Source: CAD feature listing. Evaluate the final solid. Frame: model axes, mm. Give positions to 0.01 mm unless a question says otherwise; leave off trailing zeros. Order: outer loops, then holes, each group sorted by start corner. A loop starts at its lowest first (then second) coordinate and runs counter-clockwise, first axis right, second up. Notation, with made-up numbers: (-5.75, -7.5) - (9.25, -7.5) arc R18 ccw to (9.25, 1.5) - close; hole circle Ø1 at (46, 44). An arc over 180 degrees is marked (long way). Use CSV: the item, a comma, the result in double quotes.
```python
from build123d import *

# Parameters (mm, degrees)
SKETCH_1_W          = 70
SKETCH_1_H          = 133.34
EXTRUDE_1_DEPTH     = 1.6
SKETCH_2_R          = 1.5
SKETCH_2_W          = 18
SKETCH_2_H          = 1
SKETCH_2_W_2        = 17.5
SKETCH_2_W_3        = 7.5
CUT_EXTRUDE_1_DEPTH = 76.315661718
FILLET_1_R          = 3
FILLET_2_R          = 0.5


with BuildPart() as part:
    # ｽｹｯﾁ1 → ﾎﾞｽ - 押し出し1 (new body)
    with BuildSketch(Plane(origin=(0, 0, 0), x_dir=(1, 0, 0), z_dir=(0, 1, 0))):
        Rectangle(SKETCH_1_W, SKETCH_1_H)
    extrude(amount=EXTRUDE_1_DEPTH)

    # ｽｹｯﾁ2 → ｶｯﾄ - 押し出し1 (cut, through all)
    with BuildSketch(Plane(origin=(0, 1.6, 0), x_dir=(1, 0, 0), z_dir=(0, 1, 0))):
        with Locations(Location((-22.86, -37.46, 0), (0, 0, 270))):
            Circle(SKETCH_2_R)
        with Locations(Location((22.86, -37.46, 0), (0, 0, 90))):
            Circle(SKETCH_2_R)
        with Locations(Location((-24.13, 41.65, 0), (0, 0, 270))):
            Circle(SKETCH_2_R)
        with Locations(Location((24.13, 39.95, 0), (0, 0, 270))):
            Circle(SKETCH_2_R)
        with Locations(Location((8.89, -10.85, 0), (0, 0, 270))):
            Circle(SKETCH_2_R)
        with Locations((-26, 44.15)):
            Rectangle(SKETCH_2_W, SKETCH_2_H)
        with Locations((26, 44.15)):
            Rectangle(SKETCH_2_W, SKETCH_2_H)
        with Locations((-5.25, 44.15)):
            Rectangle(SKETCH_2_W_2, SKETCH_2_H)
        with Locations((10.25, 44.15)):
            Rectangle(SKETCH_2_W_3, SKETCH_2_H)
    extrude(amount=-CUT_EXTRUDE_1_DEPTH, mode=Mode.SUBTRACT)

    # ﾌｨﾚｯﾄ1
    fillet_1_edges = [part.edges().sort_by_distance(p)[0] for p in [
        (35, 0.8, 66.67),
        (-35, 0.8, 66.67),
        (-35, 0.8, -66.67),
        (35, 0.8, -66.67),
    ]]
    fillet(fillet_1_edges, radius=FILLET_1_R)

    # ﾌｨﾚｯﾄ2
    fillet_2_edges = [part.edges().sort_by_distance(p)[0] for p in [
        (17, 0.8, -44.65),
        (17, 0.8, -43.65),
        (14, 0.8, -43.65),
        (14, 0.8, -44.65),
        (6.5, 0.8, -44.65),
        (6.5, 0.8, -43.65),
        (3.5, 0.8, -43.65),
        (3.5, 0.8, -44.65),
        (-17, 0.8, -44.65),
        (-17, 0.8, -43.65),
        (-14, 0.8, -43.65),
        (-14, 0.8, -44.65),
    ]]
    fillet(fillet_2_edges, radius=FILLET_2_R - 0.0001)  # a hair under: the kernel refuses the full size


solid = part.part
```
Item 1: Section B-B on x = 8.89. Return the cut outline in (y, z), then the cut area to 3 significant figures.
Filled in:
outline,"(0, -66.67) - (1.6, -66.67) - (1.6, -44.65) - (0, -44.65) - close; (0, -43.65) - (1.6, -43.65) - (1.6, 9.35) - (0, 9.35) - close; (0, 12.35) - (1.6, 12.35) - (1.6, 66.67) - (0, 66.67) - close"
area,"207 mm2"
Item 2: Section A-A on z = 10.85. Return the cut outline in (x, y).
Filled in:
outline,"(-35, 0) - (7.39, 0) - (7.39, 1.6) - (-35, 1.6) - close; (10.39, 0) - (35, 0) - (35, 1.6) - (10.39, 1.6) - close"
Item 3: Material intervals for line 1 (X direction, y = 0.5, z = 37.46); line 2 (X direction, y = 0.7, z = -41.65); line 3 (Z direction, x = -12, y = 0.45), sorted ascending. Write a range as from..to.
Filled in:
line 1,"x = -35..-24.36, -21.36..21.36, 24.36..35"
line 2,"x = -35..-25.63, -22.63..35"
line 3,"z = -66.67..-44.65, -43.65..66.67"
Item 4: Mould query, pull axis X, two halves, no side actions, for faces 1 (the flat face through (0, 1.6, -1)), 2 (the cylindrical face through (22.79, 0.81, 38.96)), 3 (the cylindrical face through (-25.04, 0.81, -42.84)), 4 (the cylindrical face through (34.1, 0.81, 65.81)). Classes: released by +X, released by -X, zero draft, split by the parting line, or undercut.
Filled in:
face 1,"zero draft"
face 2,"undercut"
face 3,"undercut"
face 4,"released by +X"
